Input: dimensioned drawing with shaded views. Units: mm. Origin: part minimum x, y, z. Round coordinates to 2 decimals unless told otherwise and drop trailing zeros. Loops run counter-clockwise (first coordinate to the right, second up) from the corner with the lowest first, then second, coordinate; pieces in that order, holes last. Notation, with made-up numbers: (57, 17.25) - (79, 17.25) arc R29 cw to (79, 40.25) - close; hole circle Ø6 at (80.25, -36.5). An arc over 180 degrees is marked (long way). Write each question's results on one line, items separated by ' | '.
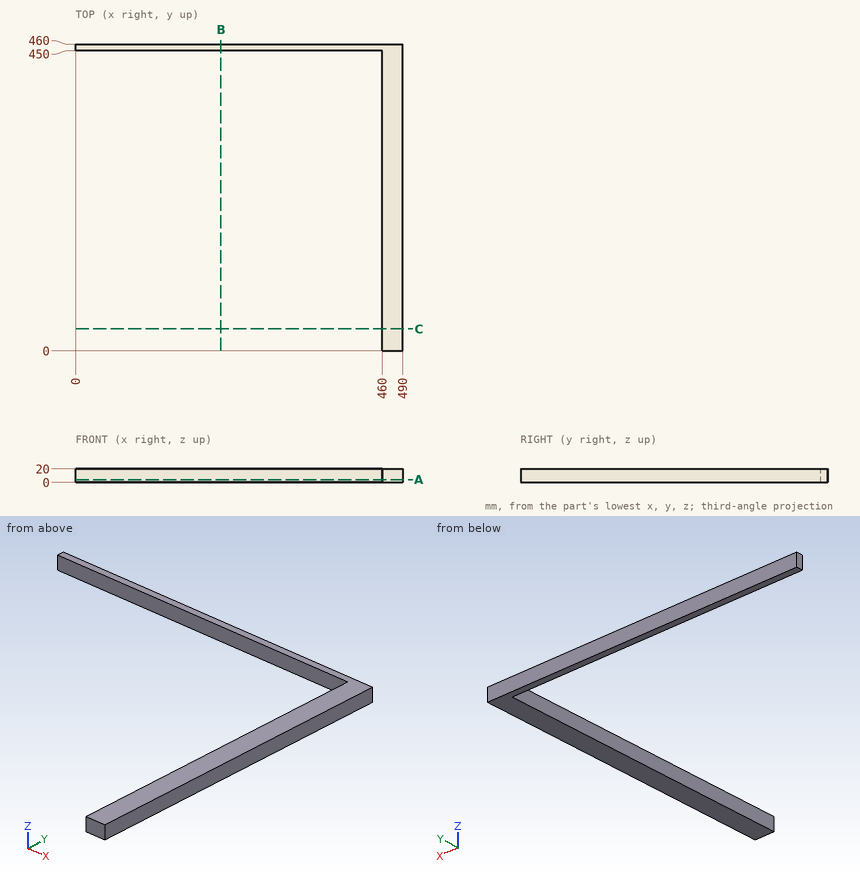
1. Section query C-C, the plane y = 33. Output: boundary loops of the cut face in (x, z).
Answer:
outline: (460, 0) - (490, 0) - (490, 20) - (460, 20) - close
2. Section query B-B, the plane x = 218. Output: boundary loops of the cut face in (y, z), plus the area to 3 significant figures.
Answer:
outline: (450, 0) - (460, 0) - (460, 20) - (450, 20) - close | area: 200 mm^2
3. Contact query for flat-ended pins moving along their axis: pin 1 (8 mm diameter, centred on x = 265.5, z = 10.5, fed in from -Y); pin 2 (1.5 mm diameter, centred on y = 175.5, z = 11.5, fed in from -X). Output: stop coordinate, or through.
Answer:
pin 1: y = 450 | pin 2: x = 460
4. Section query A-A, the plane z = 4.25. Output: boundary loops of the cut face in (x, y), plus the area to 3 significant figures.
Answer:
outline: (0, 450) - (460, 450) - (460, 0) - (490, 0) - (490, 460) - (0, 460) - close | area: 18,400 mm^2
5. Line query: line 1 (Y direction, x = 196, z = 9); line 2 (X direction, y = 240, z = 12.5). Output: solid intervals per line, ascending. Write a range as [from, to].
Answer:
line 1: [450, 460] | line 2: [460, 490]
